```python
from build123d import *

# Parameters (mm, degrees)
RESSALTO_EXTRUS_O2_DEPTH = 30
ESBO_O2_R                = 2.1
CORTE_EXTRUS_O1_DEPTH    = 63.691779646


with BuildPart() as part:
    # Esboço1 → Ressalto-extrusão2 (new body)
    with BuildSketch(Plane.XY):
        Polygon((-28.75, 15.443548387), (-28.75, -5.056451613), (-3.75, -5.056451613), (-3.75, 15.443548387), (0, 15.443548387), (0, 46.943548387), (-33.5, 46.943548387), (-33.5, 15.443548387), align=None)
        Polygon((-25, 15.443548387), (-25, -1.306451613), (-7.5, -1.306451613), (-7.5, 15.443548387), (-7.5, 16.193548387), (-25, 16.193548387), align=None, mode=Mode.SUBTRACT)
        Polygon((-25, 19.193548387), (-29.75, 19.193548387), (-29.75, 43.193548387), (-3.75, 43.193548387), (-3.75, 19.193548387), (-7.5, 19.193548387), align=None, mode=Mode.SUBTRACT)
    extrude(amount=RESSALTO_EXTRUS_O2_DEPTH)

    # Esboço2 → Corte-extrusão1 (cut, through all)
    with BuildSketch(Plane.ZY.offset(28.75)):
        with Locations(Location((15, 5.193548387, 0), (0, 0, 270))):
            Circle(ESBO_O2_R)
    extrude(amount=-CORTE_EXTRUS_O1_DEPTH, mode=Mode.SUBTRACT)


solid = part.part
```
Geometry: final body of the model. Coordinates: model frame, mm. A direction names the side the tool comes from. Give positions to 0.01 mm unless a question says otherwise; leave off trailing zeros. Loops run counter-clockwise (first coordinate to the right, second up) from the corner with the lowest first, then second, coordinate; pieces in that order, holes last. Notation, with made-up numbers: (-10, 19) - (8, 19) arc R17 cw to (8, 23) - close; hole circle Ø5 at (30, 1.5). An arc over 180 degrees is marked (long way). Answer as CSV lines item,"result". Start each with the question number.
(1) Ray query, line 1 along Y through (x, z) = (-16, 25.5); line 2 along X through (y, z) = (0.5, 8.5); line 3 along X through (y, z) = (37, 28). Return the intervals inside material, ascending. Write a range as [from, to].
(2) Pin query (flat end, axial travel): P1, Ø10, axis at y = 3, z = 13.5, coming from the -X side; P2, Ø5, axis at y = 5.19, z = 15, coming from the +X side; P3, Ø4, axis at x = -1.5, z = 7.5, coming from the -Y side. Return the tip coordinate at first contact, or that it passes through.
(3) Section query B-B (z = 15). Output: boundary loops of the cut face in (x, y).
(4) Section query D-D (x = -18). Output: boundary loops of the cut face in (y, z), and give its area (3 significant figures).
(5) Section query C-C (y = 23.5). Output: boundary loops of the cut face in (x, z).
(6) Section query A-A (x = -26). Output: boundary loops of the cut face in (y, z), and give its area (3 significant figures).
(7) Reachability of faces 1 (the face through (-6, 16, 30)), 2 (the face through (-17, 43.194, 15)), 3 (the face through (-28.75, 8, 15)), 4 (the face through (-3.75, 2.8, 14.8)) from +Z, -Z, +X, -X, +Y, -Y: full face, straight path, thin tool, end or side. Return the list, or none.
(8) Mould query, pull axis Y, two halves, no side actions, for faces 5 (the face through (-3.75, 31, 15)), 6 (the face through (-33.5, 31, 15)), 7 (the face through (-31, 15.444, 15)). Classes: +Y half, -Y half, draft (parallel to the pull), parting line (faces both ways), or undercut.
Worked answers:
1,line 1,"y = [-5.06, -1.31], [16.19, 19.19], [43.19, 46.94]"
1,line 2,"x = [-28.75, -25], [-7.5, -3.75]"
1,line 3,"x = [-33.5, -29.75], [-3.75, 0]"
2,P1,"stops at x = -28.75"
2,P2,"stops at x = -3.75"
2,P3,"stops at y = 15.44"
3,outline,"(-33.5, 15.44) - (-28.75, 15.44) - (-28.75, 7.29) - (-25, 7.29) - (-25, 16.19) - (-7.5, 16.19) - (-7.5, 7.29) - (-3.75, 7.29) - (-3.75, 15.44) - (0, 15.44) - (0, 46.94) - (-33.5, 46.94) - close; (-28.75, -5.06) - (-3.75, -5.06) - (-3.75, 3.09) - (-7.5, 3.09) - (-7.5, -1.31) - (-25, -1.31) - (-25, 3.09) - (-28.75, 3.09) - close; hole (-29.75, 19.19) - (-3.75, 19.19) - (-3.75, 43.19) - (-29.75, 43.19) - close"
4,outline,"(-5.06, 0) - (-1.31, 0) - (-1.31, 30) - (-5.06, 30) - close; (16.19, 0) - (19.19, 0) - (19.19, 30) - (16.19, 30) - close; (43.19, 0) - (46.94, 0) - (46.94, 30) - (43.19, 30) - close"
4,area,"315 mm^2"
5,outline,"(-33.5, 0) - (-29.75, 0) - (-29.75, 30) - (-33.5, 30) - close; (-3.75, 0) - (0, 0) - (0, 30) - (-3.75, 30) - close"
6,outline,"(-5.06, 0) - (19.19, 0) - (19.19, 30) - (-5.06, 30) - close; (43.19, 0) - (46.94, 0) - (46.94, 30) - (43.19, 30) - close; hole circle Ø4.2 at (5.19, 15)"
6,area,"826 mm^2"
7,face 1,"+Z, +X, -X, +Y, -Y"
7,face 2,"+Z, -Z"
7,face 3,"+Z, -Z, -X, -Y"
7,face 4,"+Z, -Z, +X, -Y"
8,face 5,"undercut"
8,face 6,"draft"
8,face 7,"-Y half"
